Check sheet for the modelled part. Datum: model origin and axes. Units: mm. Face numbers are marked on the shaded views. Give positions to 0.01 mm unless a question says otherwise; leave off trailing zeros. Write each loop counter-clockwise with the first axis right and the second up, starting at its lowest first coordinate (ties: lowest second). Pieces come first, ordered by that corner, then holes.
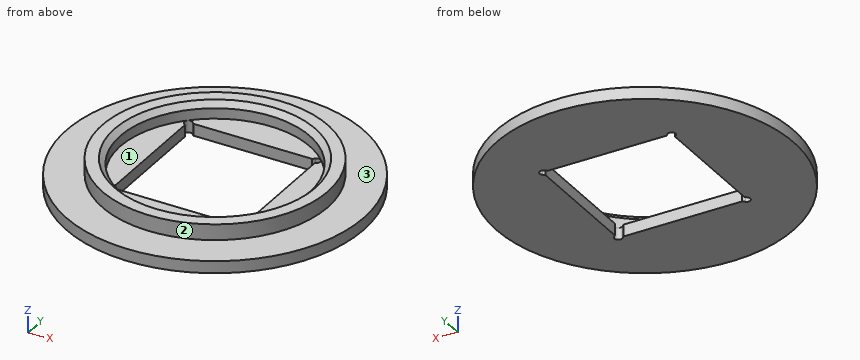
from build123d import *

# Parameters (mm, degrees)
SKETCH_1_R          = 8
EXTRUDE_1_DEPTH     = 0.65
EXTRUDE_START       = 0.65
SKETCH_2_R          = 6.07
SKETCH_2_R_2        = 5.1
EXTRUDE_2_DEPTH     = 0.85
CUT_EXTRUDE_START   = 0.65
SKETCH_3_R          = 5.1
CUT_EXTRUDE_1_DEPTH = 0.01
CUT_EXTRUDE_2_DEPTH = 0.64
CHAMFER_1_SIZE      = 0.3
SKETCH_6_R          = 0.207363545
CUT_EXTRUDE_3_DEPTH = 0.64
CUT_EXTRUDE_4_DEPTH = 0.64


with BuildPart() as part:
    # 草图1 → 凸台-拉伸1 (new body)
    with BuildSketch(Plane.XY):
        Circle(SKETCH_1_R)
    extrude(amount=EXTRUDE_1_DEPTH)

    # 草图2 → 凸台-拉伸2 (add)
    with BuildSketch(Plane.XY.offset(EXTRUDE_START)):
        Circle(SKETCH_2_R)
        Circle(SKETCH_2_R_2, mode=Mode.SUBTRACT)
    extrude(amount=EXTRUDE_2_DEPTH)

    # 草图3 → 切除-拉伸1 (cut)
    with BuildSketch(Plane.XY.offset(CUT_EXTRUDE_START)):
        Circle(SKETCH_3_R)
    extrude(amount=-CUT_EXTRUDE_1_DEPTH, mode=Mode.SUBTRACT)

    # 草图4 → 切除-拉伸2 (cut)
    with BuildSketch(Plane.XY):
        Polygon((-3.49, 0), (-3.49, 3.49), (3.49, 3.49), (3.49, -3.49), (-3.49, -3.49), align=None)
    extrude(amount=CUT_EXTRUDE_2_DEPTH, mode=Mode.SUBTRACT)

    # 倒角1
    chamfer_1_edges = [part.edges().sort_by_distance(p)[0] for p in [
        (-5.1, 0, 1.5),
    ]]
    chamfer(chamfer_1_edges, length=CHAMFER_1_SIZE)

    # 草图6 → 切除-拉伸3 (cut)
    with BuildSketch(Plane.XY):
        with Locations((-3.45, 3.45)):
            Circle(SKETCH_6_R)
        with Locations((3.45, 3.45)):
            Circle(SKETCH_6_R)
        with Locations((3.45, -3.45)):
            Circle(SKETCH_6_R)
        with Locations((-3.45, -3.45)):
            Circle(SKETCH_6_R)
    extrude(amount=CUT_EXTRUDE_3_DEPTH, mode=Mode.SUBTRACT)

    # 草图7 → 切除-拉伸4 (cut)
    with BuildSketch(Plane.XY):
        Polygon((-3.45, 3.45), (-3.596628169, 3.303371831), (-3.126421006, 2.833164668), (-2.833164668, 3.126421006), (-3.303371831, 3.596628169), align=None)
        Polygon((2.833164668, 3.126421006), (3.126421006, 2.833164668), (3.596628169, 3.303371831), (3.45, 3.45), (3.303371831, 3.596628169), align=None)
        Polygon((3.45, -3.45), (3.596628169, -3.303371831), (3.126421006, -2.833164668), (2.833164668, -3.126421006), (3.303371831, -3.596628169), align=None)
        Polygon((-2.833164668, -3.126421006), (-3.126421006, -2.833164668), (-3.596628169, -3.303371831), (-3.45, -3.45), (-3.303371831, -3.596628169), align=None)
    extrude(amount=CUT_EXTRUDE_4_DEPTH, mode=Mode.SUBTRACT)


solid = part.part
1) Scan lines: L1, parallel to Y at x = 0, z = 0.9; L2, parallel to Z at x = 6.75, y = 3.5; L3, parallel to Y at x = 3.25, z = 1. Record each from-to range of solid material in increasing order.
2) Sectioned sample at C-C on z = 0.35. Record the boundary of the cut face in (x, y).
3) Gauge pin test, flat end, axial feed: pin 1 (0.7 mm diameter, centred on y = 1.5, z = 0.5, fed in from -X). Record the tip position at first contact, or that the pin passes through.
4) Draft check along Y on the marked faces 1, 2 and 3. Enter one of: +Y half, -Y half, draft (parallel to the pull), parting line (faces both ways), or undercut.
5) Sectioned sample at D-D on y = 7.25. Record the boundary of the cut face in (x, z).
6) Sectioned sample at A-A on x = 0. Record the boundary of the cut face in (y, z), then the cut area to 3 significant figures.
Answers below:
1. L1: y = -6.07 to -5.1, 5.1 to 6.07
1. L2: z = 0 to 0.65
1. L3: y = -5.13 to -3.93, 3.93 to 5.13
2. outline: circle Ø16 at (0, 0); hole (-3.6, -3.3) arc R0.21 ccw to (-3.3, -3.6) - (-3.2, -3.49) - (3.2, -3.49) - (3.3, -3.6) arc R0.21 ccw to (3.6, -3.3) - (3.49, -3.2) - (3.49, 3.2) - (3.6, 3.3) arc R0.21 ccw to (3.3, 3.6) - (3.2, 3.49) - (-3.2, 3.49) - (-3.3, 3.6) arc R0.21 ccw to (-3.6, 3.3) - (-3.49, 3.2) - (-3.49, -3.2) - close
3. pin 1: stops at x = -7.92
4. face 1: undercut
4. face 2: parting line
4. face 3: draft
5. outline: (-3.38, 0) - (3.38, 0) - (3.38, 0.65) - (-3.38, 0.65) - close
6. outline: (-8, 0) - (-3.49, 0) - (-3.49, 0.64) - (-5.1, 0.64) - (-5.1, 1.2) - (-5.4, 1.5) - (-6.07, 1.5) - (-6.07, 0.65) - (-8, 0.65) - close; (3.49, 0) - (8, 0) - (8, 0.65) - (6.07, 0.65) - (6.07, 1.5) - (5.4, 1.5) - (5.1, 1.2) - (5.1, 0.64) - (3.49, 0.64) - close
6. area: 7.39 mm2
